```python
from build123d import *

# Parameters (mm, degrees)
SKETCH1_W                       = 115
SKETCH1_H                       = 30
EXTRUDE1_DEPTH                  = 1
SKETCH2_R                       = 1.5
MOUNT_HOLES_CUT_DEPTH           = 1
SKETCH4_W                       = 13.516297105
SKETCH4_H                       = 8.221252878
SKETCH4_W_2                     = 14.631043257
INDUCTORS_DEPTH                 = 5.5
SKETCH5_W                       = 6.291348601
SKETCH5_H                       = 15.467102872
SKETCH5_W_2                     = 7.96346783
SKETCH5_H_2                     = 16.999878832
CCFL_CONN_DEPTH                 = 5
SKETCH6_W                       = 14.156835531
SKETCH6_H                       = 4.690856218
MATE_AND_WIRE_STICK_OUT_1_DEPTH = 5.08
SKETCH7_W                       = 14.117118553
SKETCH7_H                       = 3.532074628
MATE_AND_WIRE_STICK_OUT_2_DEPTH = 5.08


with BuildPart() as part:
    # Sketch1 → Extrude1 (new body)
    with BuildSketch(Plane(origin=(0, 0, 0), x_dir=(1, 0, 0), z_dir=(0, 1, 0))):
        with Locations((57.5, -15)):
            Rectangle(SKETCH1_W, SKETCH1_H)
    extrude(amount=EXTRUDE1_DEPTH)

    # Sketch2 → mount holes - cut (cut)
    with BuildSketch(Plane(origin=(0, 1, 0), x_dir=(-1, 0, 0), z_dir=(0, 1, 0))):
        with Locations((-109, 4)):
            Circle(SKETCH2_R)
        with Locations((-6, 26)):
            Circle(SKETCH2_R)
    extrude(amount=-MOUNT_HOLES_CUT_DEPTH, mode=Mode.SUBTRACT)

    # Sketch4 → inductors (add)
    with BuildSketch(Plane(origin=(0, 1, 0), x_dir=(-1, 0, 0), z_dir=(0, 1, 0))):
        with Locations((-86.204713438, 13.606567309)):
            Rectangle(SKETCH4_W, SKETCH4_H)
        with Locations((-25.172361566, 13.606567309)):
            Rectangle(SKETCH4_W_2, SKETCH4_H)
    extrude(amount=INDUCTORS_DEPTH)

    # Sketch5 → ccfl conn (add)
    with BuildSketch(Plane(origin=(0, 1, 0), x_dir=(-1, 0, 0), z_dir=(0, 1, 0))):
        with Locations((-111.8543257, 17.647522113)):
            Rectangle(SKETCH5_W, SKETCH5_H)
        with Locations((-3.981733915, 12.143462983)):
            Rectangle(SKETCH5_W_2, SKETCH5_H_2)
    extrude(amount=CCFL_CONN_DEPTH)

    # Sketch6 → mate and wire stick-out 1 (add)
    with BuildSketch(Plane(origin=(115, 0, 0), x_dir=(0, 0, -1), z_dir=(1, 0, 0))):
        with Locations((-17.7667625, 2.941021447)):
            Rectangle(SKETCH6_W, SKETCH6_H)
    extrude(amount=MATE_AND_WIRE_STICK_OUT_1_DEPTH)

    # Sketch7 → mate and wire stick-out 2 (add)
    with BuildSketch(Plane.ZY):
        with Locations((11.841645931, 2.849567483)):
            Rectangle(SKETCH7_W, SKETCH7_H)
    extrude(amount=MATE_AND_WIRE_STICK_OUT_2_DEPTH)


solid = part.part
```
Work out the finished part from the listing and answer in its coordinate system (mm). A direction names the side the tool comes from. Coordinates: 2 decimals unless noted, no trailing zeros. Write each loop counter-clockwise with the first axis right and the second up, starting at its lowest first coordinate (ties: lowest second). Pieces come first, ordered by that corner, then holes. Notation, with made-up numbers: (47.25, -21.75) - (56.25, -21.75) arc R20 ccw to (56.25, -14.75) - close; hole circle Ø7 at (42.5, 67.5). An arc over 180 degrees is marked (long way). Answer as a JSON object with one key per item and string values.
Q1. Consider L1, parallel to X at y = 3.75, z = 12.25; L2, parallel to Z at x = 6, y = 0.3; L3, parallel to Z at x = 109, y = 0.7. Determine where each line is inside the solid, lowest interval first. Write a range as from..to.
Results list:
{"L1": "x = -5.08..7.96, 17.86..32.49, 79.45..92.96, 108.71..120.08", "L2": "z = 0..24.5, 27.5..30", "L3": "z = 0..2.5, 5.5..30"}
Q2. Find section A-A (x = 6). Write down the section's boundary in (y, z).
Results list:
{"outline": "(0, 0) - (1, 0) - (1, 3.64) - (6, 3.64) - (6, 20.64) - (1, 20.64) - (1, 24.5) - (0, 24.5) - close; (0, 27.5) - (1, 27.5) - (1, 30) - (0, 30) - close"}
Q3. Find section C-C (z = 12). Write down the section's boundary in (x, y), plus the area to 3 significant figures.
Results list:
{"outline": "(-5.08, 1.08) - (0, 1.08) - (0, 0) - (115, 0) - (115, 0.6) - (120.08, 0.6) - (120.08, 5.29) - (115, 5.29) - (115, 6) - (108.71, 6) - (108.71, 1) - (92.96, 1) - (92.96, 6.5) - (79.45, 6.5) - (79.45, 1) - (32.49, 1) - (32.49, 6.5) - (17.86, 6.5) - (17.86, 1) - (7.96, 1) - (7.96, 6) - (0, 6) - (0, 4.62) - (-5.08, 4.62) - close", "area": "383 mm^2"}
Q4. For a pull along X with two mould halves and no side action, classify faces 4 (the cylindrical face through (110.5, 0.51, 4.07)), 5 (the flat face through (79.447, 4, 14)), 6 (the flat face through (4, 3, 3.644)), 7 (the flat face through (-5.08, 3, 12)) as pulls with the +X half, pulls with the -X half, needs draft (parallel to the pull), parting line crosses it, or undercut.
Results list:
{"face 4": "undercut", "face 5": "undercut", "face 6": "needs draft", "face 7": "pulls with the -X half"}
Q5. Find section B-B (y = 3.5). Write down the section's boundary in (x, z), plus the area to 3 significant figures.
Results list:
{"outline": "(-5.08, 4.78) - (0, 4.78) - (0, 3.64) - (7.96, 3.64) - (7.96, 20.64) - (0, 20.64) - (0, 18.9) - (-5.08, 18.9) - close; (17.86, 9.5) - (32.49, 9.5) - (32.49, 17.72) - (17.86, 17.72) - close; (79.45, 9.5) - (92.96, 9.5) - (92.96, 17.72) - (79.45, 17.72) - close; (108.71, 9.91) - (115, 9.91) - (115, 10.69) - (120.08, 10.69) - (120.08, 24.85) - (115, 24.85) - (115, 25.38) - (108.71, 25.38) - close", "area": "608 mm^2"}
Q6. Given pin 1 Ø1 at (x, z) = (72.5, 10.5) entering from +Y; pin 2 Ø2 at (x, y) = (31.5, 5.5) entering from -Z; pin 3 Ø1.9 at (x, z) = (113, 20) entering from +Y, each flat-ended and moving along its own axis, determine where each tip first touches the part or whether it passes through.
Results list:
{"pin 1": "stops at y = 1", "pin 2": "stops at z = 9.5", "pin 3": "stops at y = 6"}
Q7. Which of the six approach directions +Z, -Z, +X, -X, +Y, -Y give full straight-line access (tool end or side, diameter ignored) to faces 1 (the flat face through (25, 4, 17.717)), 2 (the flat face through (118, 5.286, 18)), 3 (the flat face through (25, 4, 9.496))?
Results list:
{"face 1": "+Z, +Y", "face 2": "+Z, -Z, +X, +Y", "face 3": "-Z, +X, +Y"}
Q8. Find section D-D (x = 27.5). Write down the section's boundary in (y, z).
Results list:
{"outline": "(0, 0) - (1, 0) - (1, 9.5) - (6.5, 9.5) - (6.5, 17.72) - (1, 17.72) - (1, 30) - (0, 30) - close"}
